Source: three-view drawing plus pictorial views. Frame: mm from the lowest corner of the part. A direction names the side the tool comes from. Give positions to 0.01 mm unless a question says otherwise; leave off trailing zeros. Loops run counter-clockwise (first coordinate to the right, second up) from the corner with the lowest first, then second, coordinate; pieces in that order, holes last. Notation, with made-up numbers: (68, -17) -> (87, -17) arc R29 cw to (87, 19) -> close; hole circle Ø10 at (-13, -2.75). An arc over 180 degrees is marked (long way). Answer as a JSON object with one key per item and string values. Group by question number.
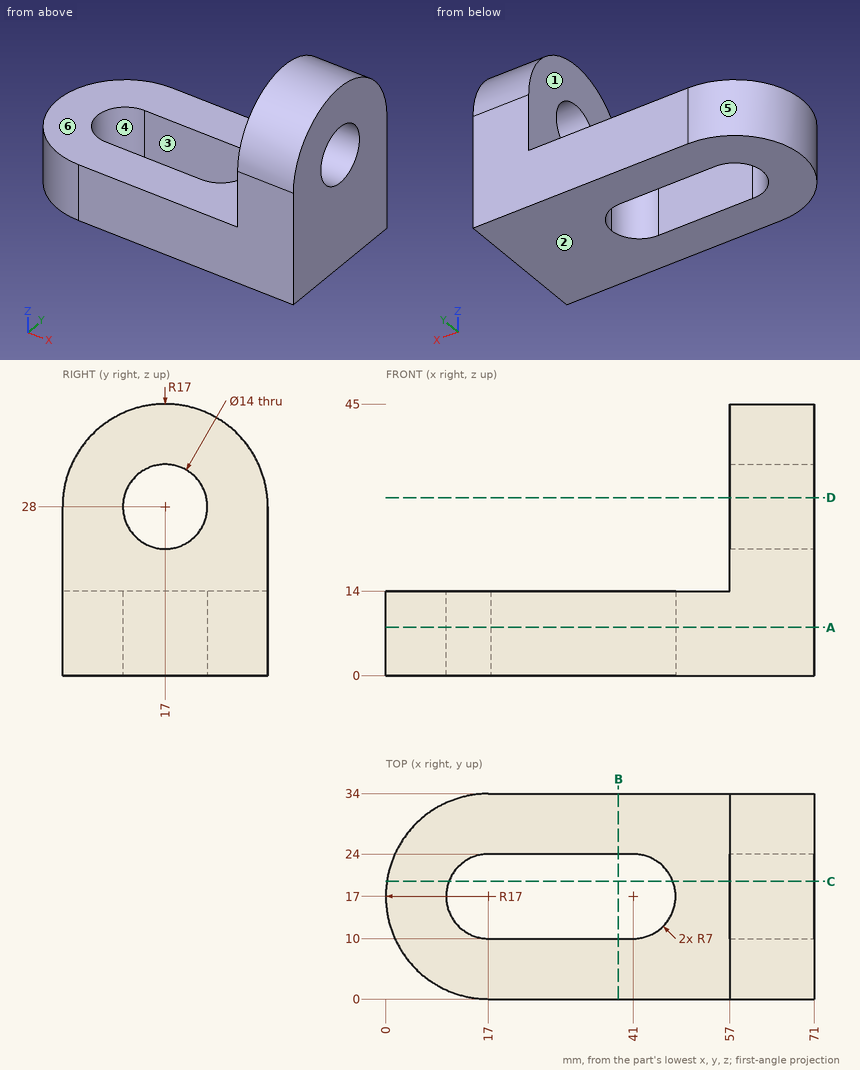
Q1. Section A-A on z = 8. Return the cut outline in (x, y).
Q2. Set-up query: the marked faces 1, 2 and 3. Return all of +Z, -Z, +X, -X, +Y, -Y with unobstructed straight access to the full face (end or side cutting, diameter ignored); none if empty.
Q3. Section D-D on z = 29.5. Return the cut outline in (x, y).
Q4. Ray query, probe 1 along Z at (x, y) = (61.75, 17); probe 2 along X at (y, z) = (5.5, 24); probe 3 along X at (y, z) = (19.5, 3). Return the intervals inside material, ascending.
Q5. Pin query (flat end, axial travel): pin 1 Ø18 at (y, z) = (17, 28) entering from -X; pin 2 Ø10 at (x, y) = (51.5, 3.5) entering from +Z; pin 3 Ø5 at (x, y) = (61.5, 12.5) entering from -Z. Return the tip coordinate at first contact, or that it passes through.
Q6. Pull-direction query (X, two-part tool) for the marked faces 4, 5 and 6; classes: +X half, -X half, draft (parallel to the pull), parting line (faces both ways), or undercut.
Q7. Section B-B on x = 38.5. Return the cut outline in (y, z), then the cut area to 3 significant figures.
Q8. Section C-C on y = 19.5. Return the cut outline in (x, z).
Numbers:
{
 "1": {"outline": "(17, 0) -> (71, 0) -> (71, 34) -> (17, 34) arc R17 ccw to start; hole (17, 24) arc R7 ccw (long way) to (17.36, 10.01) -> (41, 10) arc R7 ccw to (41, 24) -> close"},
 "2": {"face 1": "+Z, -X, +Y, -Y", "face 2": "-Z, +X, -X, +Y, -Y", "face 3": "+Z, -Z"},
 "3": {"outline": "(57, 0.07) -> (71, 0.07) -> (71, 10.16) -> (57, 10.16) -> close; (57, 23.84) -> (71, 23.84) -> (71, 33.93) -> (57, 33.93) -> close"},
 "4": {"probe 1": "z = 0 to 21, 35 to 45", "probe 2": "x = 57 to 71", "probe 3": "x = 0.18 to 10.46, 47.54 to 71"},
 "5": {"pin 1": "stops at x = 57", "pin 2": "stops at z = 14", "pin 3": "stops at z = 0"},
 "6": {"face 4": "undercut", "face 5": "-X half", "face 6": "draft"},
 "7": {"outline": "(0, 0) -> (10, 0) -> (10, 14) -> (0, 14) -> close; (24, 0) -> (34, 0) -> (34, 14) -> (24, 14) -> close", "area": "280 mm²"},
 "8": {"outline": "(0.18, 0) -> (10.46, 0) -> (10.46, 14) -> (0.18, 14) -> close; (47.54, 0) -> (71, 0) -> (71, 21.46) -> (57, 21.46) -> (57, 14) -> (47.54, 14) -> close; (57, 34.54) -> (71, 34.54) -> (71, 44.82) -> (57, 44.82) -> close"}
}
